Here's how the part is built. I have some questions about the finished solid (model axes, mm). Face numbers are marked on the shaded views. Round coordinates to 2 decimals unless told otherwise and drop trailing zeros. Order: outer loops, then holes, each group sorted by start corner. A loop starts at its lowest first (then second) coordinate and runs counter-clockwise, first axis right, second up. Notation, with made-up numbers: (4.25, 57) - (53.25, 57) arc R15 cw to (53.25, 66) - close; hole circle Ø6 at (85.25, 18). An arc over 180 degrees is marked (long way). Answer as a JSON object with one key per item and string values.
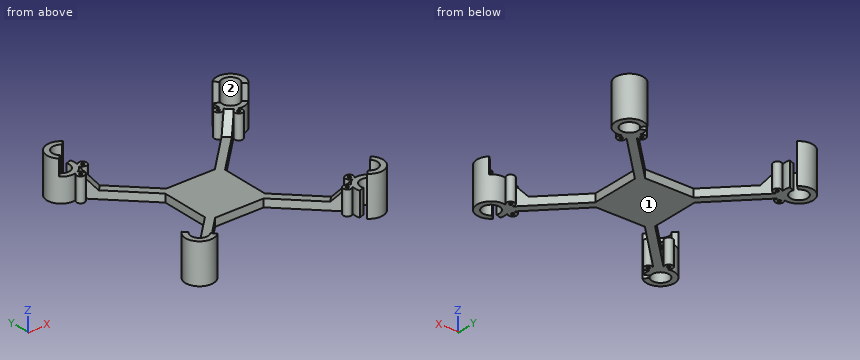
```python
from build123d import *

# Parameters (mm, degrees)
RESSALTO_EXTRUS_O1_DEPTH = 4
RESSALTO_EXTRUS_O2_DEPTH = 20
CHANFRO1_SIZE            = 8
CORTE_EXTRUS_O1_DEPTH    = 8
RESSALTO_EXTRUS_O3_START = -12
ESBO_O3_R                = 0.7499999999999987
ESBO_O3_R_2              = 0.7499999999999968
ESBO_O3_R_3              = 0.7500000000000008
ESBO_O3_R_4              = 0.7500000000000033
ESBO_O3_R_5              = 0.7499999999999941
RESSALTO_EXTRUS_O3_DEPTH = 12


with BuildPart() as part:
    # Esboço1 → Ressalto-extrusão1 (new body)
    with BuildSketch(Plane.XY):
        with BuildLine():
            ThreePointArc((39.17079707212046, 36.342369947374344), (37.5502525316941, 37.55025253169418), (36.342369947374266, 39.17079707212054))
            Line((36.342369947374266, 39.17079707212054), (12.171572875253798, 15))
            Line((12.171572875253798, 15), (-12.171572875253808, 15))
            Line((-12.171572875253808, 15), (-36.342369947374394, 39.17079707212054))
            ThreePointArc((-36.342369947374394, 39.17079707212054), (-37.55025253169423, 37.550252531694184), (-39.170797072120585, 36.34236994737435))
            Line((-39.1707970721206, 36.34236994737438), (-15.000000000000007, 12.171572875253808))
            Line((-15.000000000000007, 12.171572875253808), (-15.000000000000034, -12.171572875253805))
            Line((-15.000000000000034, -12.171572875253805), (-39.1707970721206, -36.34236994737438))
            ThreePointArc((-39.170797072120585, -36.34236994737435), (-37.55025253169423, -37.550252531694184), (-36.342369947374394, -39.17079707212054))
            Line((-36.342369947374394, -39.17079707212054), (-12.171572875253837, -14.999999999999996))
            Line((-12.171572875253837, -14.999999999999996), (12.171572875253744, -14.999999999999996))
            Line((12.171572875253743, -14.999999999999996), (36.342369947374266, -39.17079707212054))
            ThreePointArc((36.342369947374266, -39.17079707212054), (37.5502525316941, -37.55025253169418), (39.17079707212046, -36.342369947374344))
            Line((39.17079707212048, -36.34236994737438), (14.99999999999994, -12.171572875253805))
            Line((14.99999999999994, -12.171572875253805), (14.999999999999996, 12.171572875253808))
            Line((14.999999999999996, 12.171572875253808), (39.17079707212048, 36.34236994737438))
        make_face()
    extrude(amount=RESSALTO_EXTRUS_O1_DEPTH)

    # Esboço1<4> → Ressalto-extrusão2 (add)
    with BuildSketch(Plane.XY):
        with BuildLine():
            Line((-38.506306361659945, 43.95358560913411), (-35.92215165449871, 44.8941410032797))
            ThreePointArc((-35.92215165449871, 44.8941410032797), (-35.51879172736745, 41.98742702556037), (-36.342369947374394, 39.17079707212054))
            ThreePointArc((-36.342369947374394, 39.17079707212054), (-49.42666685814673, 41.489412924952944), (-37.5502525316942, 47.449747468305816))
            Line((-37.5502525316942, 47.449747468305816), (-39.49479617995721, 45.50520382004282))
            ThreePointArc((-39.49479617995721, 45.50520382004282), (-46.08441364470481, 40.216476664526006), (-38.506306361659945, 43.95358560913411))
        make_face()
        with BuildLine():
            ThreePointArc((36.342369947374266, 39.17079707212054), (49.426666858146646, 41.48941292495294), (37.550252531694085, 47.449747468305816))
            Line((37.550252531694085, 47.449747468305816), (39.494796179957106, 45.50520382004282))
            ThreePointArc((39.494796179957106, 45.50520382004282), (46.08441364470471, 40.216476664526006), (38.50630636165983, 43.95358560913411))
            Line((38.50630636165983, 43.95358560913411), (35.922151654498585, 44.8941410032797))
            ThreePointArc((35.922151654498585, 44.8941410032797), (35.51879172736732, 41.98742702556037), (36.342369947374266, 39.17079707212054))
        make_face()
        with BuildLine():
            ThreePointArc((35.922151654498585, -44.8941410032797), (35.51879172736732, -41.98742702556037), (36.342369947374266, -39.17079707212054))
            ThreePointArc((36.342369947374266, -39.17079707212054), (49.426666858146646, -41.48941292495294), (37.550252531694085, -47.449747468305816))
            Line((37.550252531694085, -47.449747468305816), (39.494796179957106, -45.50520382004282))
            ThreePointArc((39.494796179957106, -45.50520382004282), (46.08441364470471, -40.216476664526006), (38.50630636165983, -43.95358560913411))
            Line((38.50630636165983, -43.95358560913411), (35.922151654498585, -44.8941410032797))
        make_face()
        with BuildLine():
            ThreePointArc((-35.92215165449871, -44.8941410032797), (-35.51879172736745, -41.98742702556037), (-36.342369947374394, -39.17079707212054))
            ThreePointArc((-36.342369947374394, -39.17079707212054), (-49.42666685814673, -41.489412924952944), (-37.5502525316942, -47.449747468305816))
            Line((-37.5502525316942, -47.449747468305816), (-39.49479617995721, -45.50520382004282))
            ThreePointArc((-39.49479617995721, -45.50520382004282), (-46.08441364470481, -40.216476664526006), (-38.506306361659945, -43.95358560913411))
            Line((-38.506306361659945, -43.95358560913411), (-35.92215165449871, -44.8941410032797))
        make_face()
    extrude(amount=RESSALTO_EXTRUS_O2_DEPTH)

    # Chanfro1
    chanfro1_edges = [part.edges().sort_by_distance(p)[0] for p in [
        (37.5502525316941, 37.55025253169418, 4),
        (-37.55025253169423, 37.550252531694184, 4),
        (-37.55025253169423, -37.550252531694184, 4),
        (37.5502525316941, -37.55025253169418, 4),
    ]]
    chamfer(chanfro1_edges, length=CHANFRO1_SIZE)

    # Esboço2 → Corte-extrusão1 (cut)
    with BuildSketch(Plane.XY.offset(20)):
        Polygon((85.00000000000006, 0), (-2.776e-14, 85.00000000000007), (-85.00000000000007, -4.163e-14), (6.939e-14, -85.00000000000006), align=None)
    extrude(amount=-CORTE_EXTRUS_O1_DEPTH, mode=Mode.SUBTRACT)

    # Esboço3 → Ressalto-extrusão3 (add)
    # profile 1 of 8: a face of its own
    with BuildSketch(Plane(origin=(0, 0, 0), x_dir=(-1, 0, 0), z_dir=(0, 0, -1)).offset(RESSALTO_EXTRUS_O3_START)):
        with BuildLine():
            Line((38.21333643687745, 35.38490931213122), (39.17079707212057, 36.34236994737435))
            ThreePointArc((39.17079707212057, 36.34236994737435), (39.708159891817324, 36.0808389325129), (40.26587222163931, 35.866096694256335))
            ThreePointArc((40.26587222163931, 35.866096694256335), (40.08404443190525, 32.02348933210357), (38.21333643687745, 35.38490931213122))
        make_face()
        with Locations((39.627549999250526, 33.97069574975814)):
            Circle(ESBO_O3_R, mode=Mode.SUBTRACT)
    # profile 2 of 8: a face of its own
    with BuildSketch(Plane(origin=(0, 0, 0), x_dir=(-1, 0, 0), z_dir=(0, 0, -1)).offset(RESSALTO_EXTRUS_O3_START)):
        with BuildLine():
            Line((35.38490931213124, 38.21333643687742), (36.342369947374365, 39.17079707212055))
            ThreePointArc((36.342369947374365, 39.17079707212055), (36.08083893251292, 39.7081598918173), (35.86609669425635, 40.265872221639285))
            ThreePointArc((35.86609669425635, 40.265872221639285), (32.02348933210358, 40.08404443190522), (35.38490931213124, 38.21333643687742))
        make_face()
        with Locations((33.97069574975816, 39.6275499992505)):
            Circle(ESBO_O3_R, mode=Mode.SUBTRACT)
    # profile 3 of 8: a face of its own
    with BuildSketch(Plane(origin=(0, 0, 0), x_dir=(-1, 0, 0), z_dir=(0, 0, -1)).offset(RESSALTO_EXTRUS_O3_START)):
        with BuildLine():
            Line((35.38490931213109, -38.21333643687757), (36.342369947374216, -39.1707970721207))
            ThreePointArc((36.342369947374216, -39.1707970721207), (36.08083893251276, -39.70815989181745), (35.86609669425619, -40.265872221639434))
            ThreePointArc((35.86609669425619, -40.265872221639434), (32.023489332103416, -40.08404443190537), (35.38490931213109, -38.21333643687757))
        make_face()
        with Locations((33.970695749758, -39.62754999925065)):
            Circle(ESBO_O3_R, mode=Mode.SUBTRACT)
    # profile 4 of 8: a face of its own
    with BuildSketch(Plane(origin=(0, 0, 0), x_dir=(-1, 0, 0), z_dir=(0, 0, -1)).offset(RESSALTO_EXTRUS_O3_START)):
        with BuildLine():
            Line((38.21333643687729, -35.38490931213138), (39.17079707212043, -36.34236994737451))
            ThreePointArc((39.17079707212043, -36.34236994737451), (39.70815989181718, -36.08083893251306), (40.26587222163916, -35.866096694256484))
            ThreePointArc((40.26587222163916, -35.866096694256484), (40.08404443190512, -32.02348933210371), (38.21333643687729, -35.38490931213138))
        make_face()
        with Locations((39.627549999250384, -33.97069574975829)):
            Circle(ESBO_O3_R, mode=Mode.SUBTRACT)
    # profile 5 of 8: a face of its own
    with BuildSketch(Plane(origin=(0, 0, 0), x_dir=(-1, 0, 0), z_dir=(0, 0, -1)).offset(RESSALTO_EXTRUS_O3_START)):
        with BuildLine():
            Line((-38.2133364368777, -35.38490931213096), (-39.17079707212083, -36.34236994737408))
            ThreePointArc((-39.17079707212083, -36.34236994737408), (-39.70815989181758, -36.08083893251263), (-40.26587222163956, -35.86609669425605))
            ThreePointArc((-40.26587222163956, -35.86609669425605), (-40.08404443190547, -32.02348933210329), (-38.2133364368777, -35.38490931213096))
        make_face()
        with Locations((-39.62754999925076, -33.970695749757866)):
            Circle(ESBO_O3_R_2, mode=Mode.SUBTRACT)
    # profile 6 of 8: a face of its own
    with BuildSketch(Plane(origin=(0, 0, 0), x_dir=(-1, 0, 0), z_dir=(0, 0, -1)).offset(RESSALTO_EXTRUS_O3_START)):
        with BuildLine():
            Line((-35.384909312131505, -38.213336436877164), (-36.342369947374635, -39.170797072120294))
            ThreePointArc((-36.342369947374635, -39.170797072120294), (-36.08083893251319, -39.70815989181705), (-35.86609669425663, -40.265872221639036))
            ThreePointArc((-35.86609669425663, -40.265872221639036), (-32.02348933210386, -40.084044431905006), (-35.384909312131505, -38.213336436877164))
        make_face()
        with Locations((-33.970695749758434, -39.62754999925026)):
            Circle(ESBO_O3_R_3, mode=Mode.SUBTRACT)
    # profile 7 of 8: a face of its own
    with BuildSketch(Plane(origin=(0, 0, 0), x_dir=(-1, 0, 0), z_dir=(0, 0, -1)).offset(RESSALTO_EXTRUS_O3_START)):
        with BuildLine():
            Line((-35.38490931213082, 38.213336436877796), (-36.34236994737394, 39.17079707212094))
            ThreePointArc((-36.34236994737394, 39.17079707212094), (-36.080838932512485, 39.708159891817694), (-35.86609669425591, 40.265872221639675))
            ThreePointArc((-35.86609669425591, 40.265872221639675), (-32.02348933210314, 40.084044431905575), (-35.38490931213082, 38.213336436877796))
        make_face()
        with Locations((-33.97069574975772, 39.62754999925087)):
            Circle(ESBO_O3_R_4, mode=Mode.SUBTRACT)
    # profile 8 of 8: a face of its own
    with BuildSketch(Plane(origin=(0, 0, 0), x_dir=(-1, 0, 0), z_dir=(0, 0, -1)).offset(RESSALTO_EXTRUS_O3_START)):
        with BuildLine():
            Line((-38.21333643687705, 35.38490931213163), (-39.17079707212017, 36.34236994737476))
            ThreePointArc((-39.17079707212017, 36.34236994737476), (-39.708159891816926, 36.08083893251332), (-40.26587222163891, 35.866096694256754))
            ThreePointArc((-40.26587222163891, 35.866096694256754), (-40.0840444319049, 32.02348933210398), (-38.21333643687705, 35.38490931213163))
        make_face()
        with Locations((-39.62754999925015, 33.970695749758555)):
            Circle(ESBO_O3_R_5, mode=Mode.SUBTRACT)
    extrude(amount=RESSALTO_EXTRUS_O3_DEPTH)


solid = part.part
```
1. Imagine slicing it at A-A (x = -18). List the corners of the cut face in (y, z) for me.
Responses:
{"outline": "(-20.83, 0) - (-15.17, 0) - (-15.17, 4) - (-20.83, 4) - close; (15.17, 0) - (20.83, 0) - (20.83, 4) - (15.17, 4) - close"}
2. Thinking about a two-plate mould opening in Y: for the marked faces 1 and 2, which applies, pulls with the +Y half, pulls with the -Y half, needs draft (parallel to the pull), parting line crosses it, or undercut?
Responses:
{"face 1": "needs draft", "face 2": "undercut"}
3. Imagine slicing it at B-B (y = -16.5). List the corners of the cut face in (x, z) for me, plus the area to 3 significant figures.
Responses:
{"outline": "(-19.33, 0) - (-13.67, 0) - (-13.67, 4) - (-19.33, 4) - close; (13.67, 0) - (19.33, 0) - (19.33, 4) - (13.67, 4) - close", "area": "45.3 mm2"}
4. If I drill on L1, parallel to X at y = -42.5, z = 6.5; L2, parallel to X at y = 46, z = 8, over which ranges is the centre line in solid material (lowest first)? Write a range as [from, to].
Responses:
{"L1": "[-49.5, -46.75], [-38.25, -35.5], [35.5, 38.25], [46.75, 49.5]", "L2": "[-48.56, -44.91], [-40.09, -39], [39, 40.09], [44.91, 48.56]"}
5. For P1, Ø1.5, axis at x = -17, y = -9, coming from the +Z side; P2, Ø1.7, axis at x = -39.63, y = -33.97, coming from the +Z side; P3, Ø3, axis at y = 2, z = 2, coming from the +X side; P4, Ø4.5, axis at x = -1, z = 1.5, coming from the -Y side, each with a flat end and sliding along its axis, tell me the tip position at first contact or that it passes through.
Responses:
{"P1": "through", "P2": "z = 12", "P3": "x = 15", "P4": "y = -15"}
6. Imagine slicing it at D-D (y = -3.5). List the corners of the cut face in (x, z) for me.
Responses:
{"outline": "(-15, 0) - (15, 0) - (15, 4) - (-15, 4) - close"}
7. Imagine slicing it at C-C (z = 8). Give the number of separate pieces and of enclosed holes in the cut face, plus the area to 3 significant figures.
Responses:
{"separate pieces": "4", "enclosed holes": "8", "area": "515 mm2"}
